```python
from build123d import *

# Parameters (mm, degrees)
F0_W     = 116
F0_H     = 56
F1_DEPTH = 5
F2_R     = 1
F3_W     = 32.2175696492
F3_H     = 4.4865976088
F4_DEPTH = 10
F5_F1_R  = 2
F5_F2_R  = 2


with BuildPart() as f1:
    # F0 (on Top) → F1 (new body)
    with BuildSketch(Plane.XY):
        Rectangle(F0_W, F0_H)
    extrude(amount=F1_DEPTH)

    # F2
    f2_edges = [f1.edges().sort_by_distance(p)[0] for p in [
        (0, -28, 5),
        (-58, 0, 5),
        (0, 28, 5),
        (58, 0, 5),
    ]]
    fillet(f2_edges, radius=F2_R)

    # F3 (on face) → F4 (join)
    with BuildSketch(Plane.XY.offset(5)):
        Rectangle(F3_W, F3_H)
    extrude(amount=F4_DEPTH)

    # F5: fillet of radius 2 on 8 edges, made by hand

    # F5_f1
    f5_f1_edges = [f1.edges().sort_by_distance(p)[0] for p in [
        (-16.1087848246, -2.2432988044, 10),
        (-16.1087848246, 2.2432988044, 10),
        (0, -2.2432988044, 15),
        (0, 2.2432988044, 15),
        (16.1087848246, -2.2432988044, 10),
        (16.1087848246, 2.2432988044, 10),
    ]]
    fillet(f5_f1_edges, radius=F5_F1_R)

    # F5_f2
    f5_f2_edges = [f1.edges().sort_by_distance(p)[0] for p in [
        (0, -2.2432988044, 5),
        (0, 2.2432988044, 5),
        (15.522998387, 1.6575123668, 5),
        (-15.522998387, 1.6575123668, 5),
        (-15.522998387, -1.6575123668, 5),
        (15.522998387, -1.6575123668, 5),
    ]]
    fillet(f5_f2_edges, radius=F5_F2_R)


solid = f1.part
```
The model under review builds one solid part; all positions refer to its coordinate system, in mm. A direction names the side the tool comes from. Give positions to 0.01 mm unless a question says otherwise; leave off trailing zeros. Loops run counter-clockwise (first coordinate to the right, second up) from the corner with the lowest first, then second, coordinate; pieces in that order, holes last. Notation, with made-up numbers: (-1, 45.25) - (12, 45.25) arc R21 cw to (12, 80.25) - close; hole circle Ø2 at (-23, 37.25). An arc over 180 degrees is marked (long way). Answer as a JSON object with one key per item and string values.
Q1. Add section B-B on y = 19.5. State the section outline as (x, z) points.
Worked out:
{"outline": "(-58, 0) - (58, 0) - (58, 4) arc R1 ccw to (57, 5) - (-57, 5) arc R1 ccw to (-58, 4) - close"}
Q2. Add section A-A on x = 7. State the section outline as (y, z) points, plus the area to 3 significant figures.
Worked out:
{"outline": "(-28, 0) - (28, 0) - (28, 4) arc R1 ccw to (27, 5) - (4.24, 5) arc R2 cw to (2.24, 7) - (2.24, 13) arc R2 ccw to (0.24, 15) - (-0.24, 15) arc R2 ccw to (-2.24, 13) - (-2.24, 7) arc R2 cw to (-4.24, 5) - (-27, 5) arc R1 ccw to (-28, 4) - close", "area": "324 mm^2"}
Q3. To check wall thickness, follow line 1 along Y through (x, z) = (12, 9); line 2 along Z through (x, y) = (-24, 5.5); line 3 along Z through (x, y) = (2, 0.5). State the ranges of each line that lie inside material, in increasing order.
Worked out:
{"line 1": "y = -2.24 to 2.24", "line 2": "z = 0 to 5", "line 3": "z = 0 to 14.98"}
Q4. For faces 1 (the flat face through (0, 2.243, 10)), 2 (the cylindrical face through (-15.51, -1.67, 11.06)), 3 (the cylindrical face through (-15.51, 1.67, 11.06)), list the 3-axis set-ups (+Z, -Z, +X, -X, +Y, -Y) from which the entire face can be reached by the end or side of a thin tool; tool diameter is ignored.
Worked out:
{"face 1": "+Z, +X, -X, +Y", "face 2": "+Z, -X, -Y", "face 3": "+Z, -X, +Y"}
Q5. Add section C-C on x = 34. State the section outline as (y, z) points.
Worked out:
{"outline": "(-28, 0) - (28, 0) - (28, 4) arc R1 ccw to (27, 5) - (-27, 5) arc R1 ccw to (-28, 4) - close"}
Q6. Insertion check: pin 1 (16 mm diameter, centred on x = -24.5, y = 3, fed in from +Z); pin 2 (6 mm diameter, centred on x = -20.5, y = 7.5, fed in from +Z); pin 3 (1.8 mm diameter, centred on x = -3.5, z = 9, fed in from +Y); pin 4 (3 mm diameter, centred on x = 4.5, y = -15.5, fed in from -Z). Each pin has a flat end and moves straight along its axis. Give the tip position at first contact, or say it passes through.
Worked out:
{"pin 1": "stops at z = 5.44", "pin 2": "stops at z = 5", "pin 3": "stops at y = 2.24", "pin 4": "stops at z = 0"}
